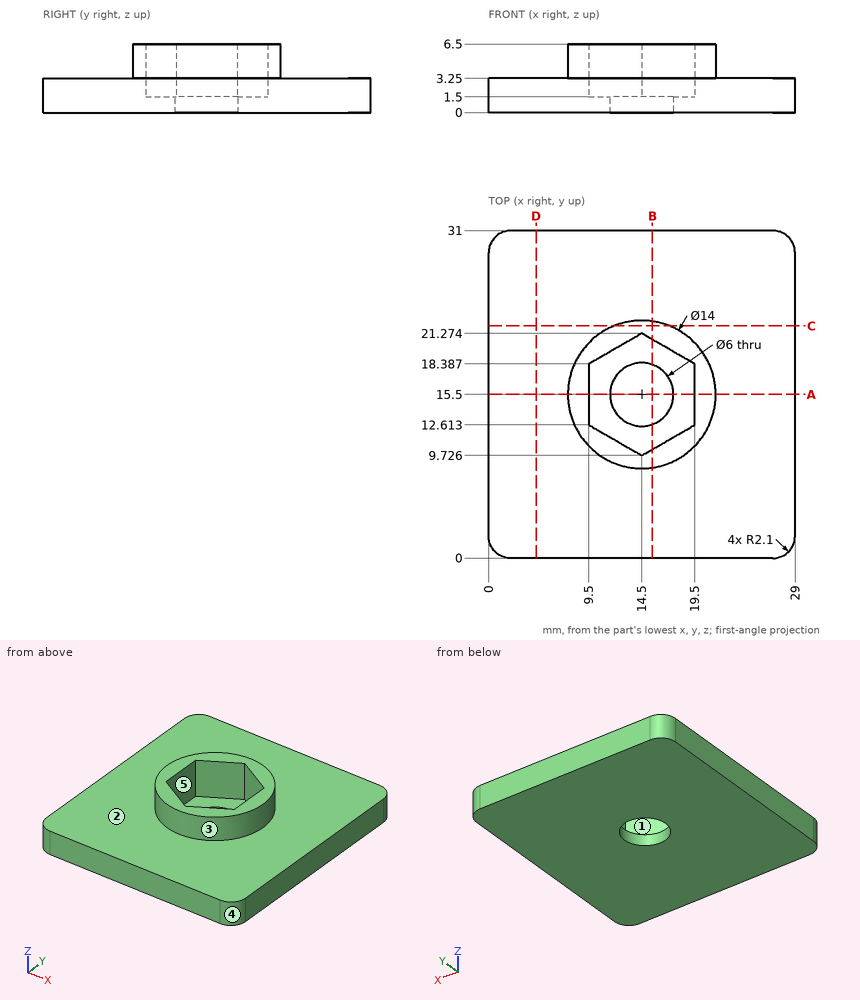
Here's the drawing with two shaded views (mm, measured from the low corner). I have some questions. A direction names the side the tool comes from. Round coordinates to 2 decimals unless told otherwise and drop trailing zeros. Order: outer loops, then holes, each group sorted by start corner. A loop starts at its lowest first (then second) coordinate and runs counter-clockwise, first axis right, second up. Notation, with made-up numbers: (-3, 0.5) -> (34, 0.5) arc R18 ccw to (34, 30.5) -> close; hole circle Ø9 at (-29.75, -4). An arc over 180 degrees is marked (long way). Return JSON: item names as keys, results as strings.
Q1. I need wall thicknesses on line 1 along X through (y, z) = (17, 2); line 2 along Y through (x, z) = (14.5, 0.3); line 3 along Z through (x, y) = (6.5, 3). Which ranges of each line are inside material? Lowest first, please. Write a range as from..to.
Filled sheet:
{"line 1": "x = 0..9.5, 19.5..29", "line 2": "y = 0..12.5, 18.5..31", "line 3": "z = 0..3.25"}
Q2. If we section it at C-C on y = 22: List the corners of the cut face in (x, z) for me.
Filled sheet:
{"outline": "(0, 0) -> (29, 0) -> (29, 3.25) -> (17.1, 3.25) -> (17.1, 6.5) -> (11.9, 6.5) -> (11.9, 3.25) -> (0, 3.25) -> close"}
Q3. If we section it at B-B on x = 15.5: List the corners of the cut face in (y, z) for me.
Filled sheet:
{"outline": "(0, 0) -> (12.67, 0) -> (12.67, 1.5) -> (10.3, 1.5) -> (10.3, 6.5) -> (8.57, 6.5) -> (8.57, 3.25) -> (0, 3.25) -> close; (18.33, 0) -> (31, 0) -> (31, 3.25) -> (22.43, 3.25) -> (22.43, 6.5) -> (20.7, 6.5) -> (20.7, 1.5) -> (18.33, 1.5) -> close"}
Q4. If we section it at A-A on y = 15.5: List the corners of the cut face in (x, z) for me.
Filled sheet:
{"outline": "(0, 0) -> (11.5, 0) -> (11.5, 1.5) -> (9.5, 1.5) -> (9.5, 6.5) -> (7.5, 6.5) -> (7.5, 3.25) -> (0, 3.25) -> close; (17.5, 0) -> (29, 0) -> (29, 3.25) -> (21.5, 3.25) -> (21.5, 6.5) -> (19.5, 6.5) -> (19.5, 1.5) -> (17.5, 1.5) -> close"}
Q5. For pin 1 Ø2 at (x, z) = (21, 4) entering from -Y; pin 2 Ø5 at (x, y) = (14.5, 15.5) entering from -Z, each with a flat end and sliding along its axis, tell me the tip position at first contact or that it passes through.
Filled sheet:
{"pin 1": "stops at y = 0", "pin 2": "passes through"}
Q6. If we mould it in two halves opening along X, with no side actions, what happens to the marked faces 1, 2 and 3? For each: released by +X, released by -X, zero draft, split by the parting line, or undercut.
Filled sheet:
{"face 1": "undercut", "face 2": "zero draft", "face 3": "split by the parting line"}
Q7. Which directions (+Z, -Z, +X, -X, +Y, -Y) give clear straight access to the entire face, cutting with the end or side of a thin tool? Please do the marked faces 4 and 5.
Filled sheet:
{"face 4": "+Z, -Z, +X, -Y", "face 5": "+Z"}
Q8. If we section it at D-D on x = 4.5: List the corners of the cut face in (y, z) for me.
Filled sheet:
{"outline": "(0, 0) -> (31, 0) -> (31, 3.25) -> (0, 3.25) -> close"}
